from build123d import *

# Parameters (mm, degrees)
SKETCH1_R           = 4
BOSS_EXTRUDE1_DEPTH = 2.5


with BuildPart() as part:
    # Sketch1 → Boss-Extrude1 (new, symmetric)
    with BuildSketch(Plane(origin=(0, 0, 0), x_dir=(0, 1, 0), z_dir=(0, 0, 1))):
        with BuildLine():
            Line((105, 14), (-105, 14))
            ThreePointArc((-105, 14), (-119, 0), (-105, -14))
            Line((-105, -14), (105, -14))
            ThreePointArc((105, -14), (119, 0), (105, 14))
        make_face()
        with Locations(Location((-105, 0, 0), (0, 0, 270))):
            Circle(SKETCH1_R, mode=Mode.SUBTRACT)
        with BuildLine():
            ThreePointArc((-2, 3.464101615), (0, 4), (2, 3.464101615))
            ThreePointArc((2, 3.464101615), (4, 4), (6, 3.464101615))
            ThreePointArc((6, 3.464101615), (10, 3.464101615), (12, 0))
            ThreePointArc((12, 0), (10, -3.464101615), (6, -3.464101615))
            ThreePointArc((6, -3.464101615), (4, -4), (2, -3.464101615))
            ThreePointArc((2, -3.464101615), (0, -4), (-2, -3.464101615))
            ThreePointArc((-2, -3.464101615), (-4, -4), (-6, -3.464101615))
            ThreePointArc((-6, -3.464101615), (-8, -4), (-10, -3.464101615))
            ThreePointArc((-10, -3.464101615), (-12, -4), (-14, -3.464101615))
            ThreePointArc((-14, -3.464101615), (-16, -4), (-18, -3.464101615))
            ThreePointArc((-18, -3.464101615), (-24, 0), (-18, 3.464101615))
            ThreePointArc((-18, 3.464101615), (-16, 4), (-14, 3.464101615))
            ThreePointArc((-14, 3.464101615), (-12, 4), (-10, 3.464101615))
            ThreePointArc((-10, 3.464101615), (-8, 4), (-6, 3.464101615))
            ThreePointArc((-6, 3.464101615), (-4, 4), (-2, 3.464101615))
        make_face(mode=Mode.SUBTRACT)
        with BuildLine():
            ThreePointArc((103, 3.464101615), (109, 0), (103, -3.464101615))
            ThreePointArc((103, -3.464101615), (101, -4), (99, -3.464101615))
            ThreePointArc((99, -3.464101615), (97, -4), (95, -3.464101615))
            ThreePointArc((95, -3.464101615), (93, -4), (91, -3.464101615))
            ThreePointArc((91, -3.464101615), (89, -4), (87, -3.464101615))
            ThreePointArc((87, -3.464101615), (85, -4), (83, -3.464101615))
            ThreePointArc((83, -3.464101615), (81, -4), (79, -3.464101615))
            ThreePointArc((79, -3.464101615), (73, 0), (79, 3.464101615))
            ThreePointArc((79, 3.464101615), (81, 4), (83, 3.464101615))
            ThreePointArc((83, 3.464101615), (85, 4), (87, 3.464101615))
            ThreePointArc((87, 3.464101615), (89, 4), (91, 3.464101615))
            ThreePointArc((91, 3.464101615), (93, 4), (95, 3.464101615))
            ThreePointArc((95, 3.464101615), (97, 4), (99, 3.464101615))
            ThreePointArc((99, 3.464101615), (101, 4), (103, 3.464101615))
        make_face(mode=Mode.SUBTRACT)
    extrude(amount=BOSS_EXTRUDE1_DEPTH, both=True)


solid = part.part
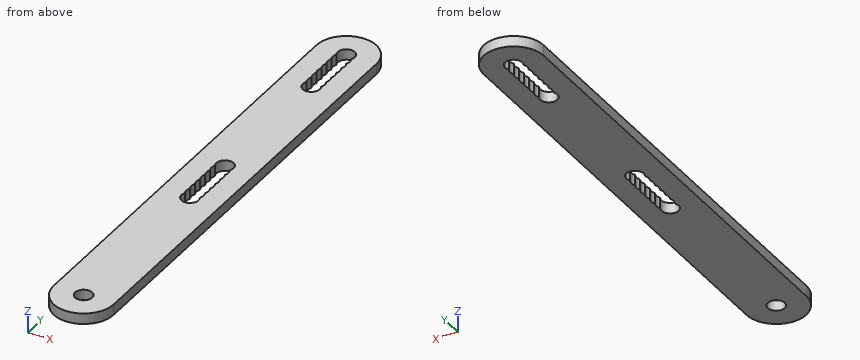
Can you work these out from the model? Positions are in its coordinate system, mm. Coordinates: 2 decimals unless noted, no trailing zeros. Write each loop counter-clockwise with the first axis right and the second up, starting at its lowest first coordinate (ties: lowest second). Pieces come first, ordered by that corner, then holes. Notation, with made-up numbers: (0.25, 24.5) -> (20.25, 24.5) arc R7 cw to (20.25, 37.5) -> close; hole circle Ø10 at (39.25, 82.5). An arc over 180 degrees is marked (long way). Write each question's results on one line, items separated by ' | '. Start each with the question number.
Item 1: If we section it at A-A, the plane z = -1.45: Count the separate pieces of the cut face and the enclosed holes in it, and give its area (3 significant figures).
Item 2: I'm going to push a flat-ended pin straight in: P1, Ø6.5, axis at x = 0, y = -20, coming from the -Z side. Where does the tip first touch, or does it pass through?
Item 3: Please list where these lines run through material, in increasing order: probe 1 along X at (y, z) = (8, 1.4); probe 2 along Y at (x, z) = (1, 0.95); probe 3 along Y at (x, z) = (-1.25, -0.8).
Item 4: If we section it at C-C, the plane y = 8: Write out the boundary of the cut face in (x, z).
Item 5: If we section it at B-B, the plane x = 0: Write out the boundary of the cut face in (y, z), and give its area (3 significant figures).
Item 6: If we section it at D-D, the plane x = 10: Write out the boundary of the cut face in (y, z).
Answer block:
1) separate pieces: 1 | enclosed holes: 3 | area: 5,920 mm²
2) P1: through
3) probe 1: -14 to -4, 4 to 14 | probe 2: -118.96 to -108.87, -101.13 to -23.87, 11.87 to 73.13, 108.87 to 118.96 | probe 3: -118.94 to -108.8, -101.2 to -23.8, 11.8 to 73.2, 108.8 to 118.94
4) outline: (-14, -2.5) -> (-4, -2.5) -> (-4, 2.5) -> (-14, 2.5) -> close; (4, -2.5) -> (14, -2.5) -> (14, 2.5) -> (4, 2.5) -> close
5) outline: (-119, -2.5) -> (-109, -2.5) -> (-109, 2.5) -> (-119, 2.5) -> close; (-101, -2.5) -> (-24, -2.5) -> (-24, 2.5) -> (-101, 2.5) -> close; (12, -2.5) -> (73, -2.5) -> (73, 2.5) -> (12, 2.5) -> close; (109, -2.5) -> (119, -2.5) -> (119, 2.5) -> (109, 2.5) -> close | area: 790 mm²
6) outline: (-114.8, -2.5) -> (114.8, -2.5) -> (114.8, 2.5) -> (-114.8, 2.5) -> close
